The model under review builds one solid part; all positions refer to its coordinate system, in mm. A direction names the side the tool comes from. Coordinates: 2 decimals unless noted, no trailing zeros. Order: outer loops, then holes, each group sorted by start corner. A loop starts at its lowest first (then second) coordinate and runs counter-clockwise, first axis right, second up.
```python
from build123d import *

# Parameters (mm, degrees)
SKETCH2_R           = 50
BOSS_EXTRUDE1_DEPTH = 360
CUT_EXTRUDE2_DEPTH  = 260


with BuildPart() as part:
    # Sketch2 → Boss-Extrude1 (new body)
    with BuildSketch(Plane.XY):
        with Locations(Location((0, 0, 0), (0, 0, 180))):
            Circle(SKETCH2_R)
    extrude(amount=BOSS_EXTRUDE1_DEPTH)

    # Sketch3 → Cut-Extrude2 (cut)
    with BuildSketch(Plane.XY):
        with BuildLine():
            Line((48.989794856, 10), (37.979794856, 10))
            Line((37.979794856, 10), (37.979794856, -10))
            Line((37.979794856, -10), (48.989794856, -10))
            ThreePointArc((48.989794856, -10), (50, 0), (48.989794856, 10))
        make_face()
    extrude(amount=CUT_EXTRUDE2_DEPTH, mode=Mode.SUBTRACT)


solid = part.part
```
(1) Wall thickness on probe 1 along Y at (x, z) = (2, 142); probe 2 along X at (y, z) = (1, 331); probe 3 along X at (y, z) = (-4, 340): over which ranges is each line inside the solid? List them lowest first.
A:
probe 1: y = -49.96 to 49.96
probe 2: x = -49.99 to 49.99
probe 3: x = -49.84 to 49.84
(2) We need section C-C, the plane x = 32.5. Write out the cut boundary in (y, z), and give its area (3 significant figures).
A:
outline: (-38, 0) - (38, 0) - (38, 360) - (-38, 360) - close
area: 27,400 mm2
(3) We need section A-A, the plane y = 0. Write out the cut boundary in (x, z), and give its area (3 significant figures).
A:
outline: (-50, 0) - (37.98, 0) - (37.98, 260) - (50, 260) - (50, 360) - (-50, 360) - close
area: 32,900 mm2
(4) We need section B-B, the plane z = 150. Write out the cut boundary in (x, y), and give its area (3 significant figures).
A:
outline: (37.98, -10) - (37.98, 10) - (48.99, 10) arc R50 ccw (long way) to (48.99, -10) - close
area: 7,620 mm2
(5) Machinability: for faces 4 (the face through (43, -10, 128)), 5 (the face through (1, -1, 360)), which of the approach directions +Z, -Z, +X, -X, +Y, -Y give a long, thin tool a straight path to every point of the face, cutting with its end or side? Answer none if there is none.
A:
face 4: -Z, +X
face 5: +Z, +X, -X, +Y, -Y
(6) Draft analysis for pull direction Y (two halves, no side actions). For faces 1 (the face through (0, -1, 0)), 2 (the face through (-47.69, -15.02, 177.48)), 3 (the face through (37.98, 0, 128)), state which applies: released by +Y, released by -Y, zero draft, split by the parting line, or undercut.
A:
face 1: zero draft
face 2: split by the parting line
face 3: undercut
(7) For pin 1 Ø8 at (x, z) = (-34, 132.5) entering from +Y; pin 2 Ø5 at (y, z) = (28.5, 308.5) entering from +X; pin 3 Ø6 at (y, z) = (4, 79.5) entering from +X, all flat-tipped, find the tip position at first contact; note any pin that passes through.
A:
pin 1: stops at y = 40
pin 2: stops at x = 42.71
pin 3: stops at x = 37.98
